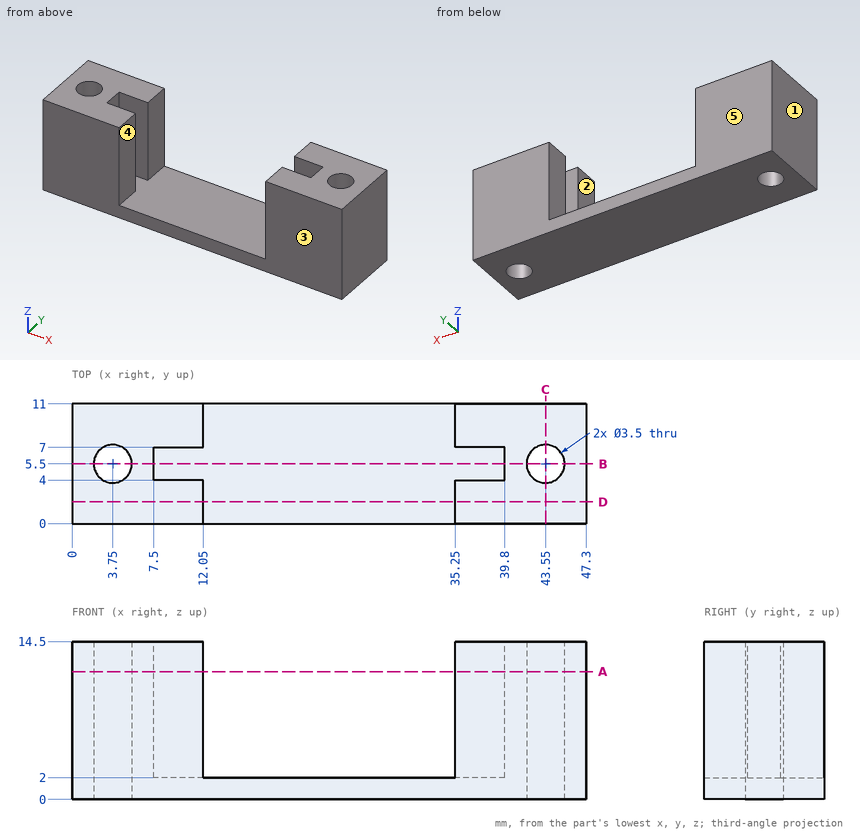
For this review, use the dimensioned drawing (mm, ordinates from the lowest corner) and the shaded views. A direction names the side the tool comes from. Round coordinates to 2 decimals unless told otherwise and drop trailing zeros. Order: outer loops, then holes, each group sorted by start corner. A loop starts at its lowest first (then second) coordinate and runs counter-clockwise, first axis right, second up.
1) Consider section B-B (y = 5.5). State the section outline as (x, z) points.
The answers:
outline: (0, 0) - (2, 0) - (2, 14.5) - (0, 14.5) - close; (5.5, 0) - (41.8, 0) - (41.8, 14.5) - (39.8, 14.5) - (39.8, 2) - (7.5, 2) - (7.5, 14.5) - (5.5, 14.5) - close; (45.3, 0) - (47.3, 0) - (47.3, 14.5) - (45.3, 14.5) - close
2) Machinability: for the marked faces 4 and 5, which of the approach directions +Z, -Z, +X, -X, +Y, -Y give a long, thin tool a straight path to every point of the face, cutting with its end or side? Answer none if there is none.
The answers:
face 4: +Z, +Y, -Y
face 5: +Z, -Z, +X, -X, +Y
3) Consider section D-D (y = 2). State the section outline as (x, z) points, plus the area to 3 significant figures.
The answers:
outline: (0, 0) - (47.3, 0) - (47.3, 14.5) - (35.25, 14.5) - (35.25, 2) - (12.05, 2) - (12.05, 14.5) - (0, 14.5) - close
area: 396 mm2
4) Clearance check with a flat-ended pin moving along its axis: pin 1 Ø3 at (x, y) = (3.75, 5.5) entering from +Z. State where the tip first meets the part, or that it passes through.
The answers:
pin 1: passes through
5) Consider section C-C (x = 43.55). State the section outline as (y, z) points, plus the area to 3 significant figures.
The answers:
outline: (0, 0) - (3.75, 0) - (3.75, 14.5) - (0, 14.5) - close; (7.25, 0) - (11, 0) - (11, 14.5) - (7.25, 14.5) - close
area: 109 mm2
6) For L1, parallel to Y at x = 3.75, z = 5; L2, parallel to X at y = 6.25, z = 11; L3, parallel to X at y = 8.5, z = 6.25, list the stretches that pass through material, from the lowest coordinate up.
The answers:
L1: y = 0 to 3.75, 7.25 to 11
L2: x = 0 to 2.17, 5.33 to 7.5, 39.8 to 41.97, 45.13 to 47.3
L3: x = 0 to 12.05, 35.25 to 47.3
7) Consider section A-A (z = 11.75). State the section outline as (x, y) points, plus the area to 3 significant figures.
The answers:
outline: (0, 0) - (12.05, 0) - (12.05, 4) - (7.5, 4) - (7.5, 7) - (12.05, 7) - (12.05, 11) - (0, 11) - close; (35.25, 0) - (47.3, 0) - (47.3, 11) - (35.25, 11) - (35.25, 7) - (39.8, 7) - (39.8, 4) - (35.25, 4) - close; hole circle Ø3.5 at (3.75, 5.5); hole circle Ø3.5 at (43.55, 5.5)
area: 219 mm2
8) Draft analysis for pull direction X (two halves, no side actions). For the marked faces 1, 2 and 3, state which applies: released by +X, released by -X, zero draft, split by the parting line, or undercut.
The answers:
face 1: released by -X
face 2: undercut
face 3: zero draft
